Model file for the job. Use its own axes, mm. Coordinates: 2 decimals unless noted, no trailing zeros. Write each loop counter-clockwise with the first axis right and the second up, starting at its lowest first coordinate (ties: lowest second). Pieces come first, ordered by that corner, then holes. Notation, with made-up numbers: M -40,39 L 2,39 A31 cw 2,71 Z; hole C -31,-31 d1. An arc over 180 degrees is marked long. Answer in a Markdown table with one row per item. Add a question column.
```python
from build123d import *

# Parameters (mm, degrees)
SKETCH1_W               = 10
SKETCH1_H               = 10
PLATE_DEPTH             = 0.5
SKETCH2_R               = 0.2
ROD_DEPTH               = 0.25
LPATTERN1_COUNT         = 10
LPATTERN1_PITCH         = 1
LPATTERN1_COUNT_DIR2    = 10
LPATTERN1_PITCH_DIR2    = 1
BOSS_EXTRUDE3_DEPTH     = 0.5
SKETCH5_R               = 1.455938962
CUT_EXTRUDE1_DEPTH      = 0.5
CUT_EXTRUDE1_DEPTH_BACK = 1.5


with BuildPart() as part:
    # Sketch1 → Plate (new body)
    with BuildSketch(Plane(origin=(0, 0, 0), x_dir=(1, 0, 0), z_dir=(0, 1, 0))):
        Rectangle(SKETCH1_W, SKETCH1_H)
    extrude(amount=PLATE_DEPTH)

    # Sketch2 → Rod (add)
    with BuildSketch(Plane(origin=(0, 0.5, 0), x_dir=(1, 0, 0), z_dir=(0, 1, 0))):
        with Locations((-4.5, -4.5)):
            Circle(SKETCH2_R)
    rod = extrude(amount=ROD_DEPTH)

    # LPattern1: Rod 10 × 10
    with Locations(*[(i * LPATTERN1_PITCH, 0, -j * LPATTERN1_PITCH_DIR2) for i in range(LPATTERN1_COUNT) for j in range(LPATTERN1_COUNT_DIR2) if (i, j) != (0, 0)]):
        add(rod)

    # Sketch4 → Boss-Extrude3 (add)
    with BuildSketch(Plane(origin=(0, 0, 0), x_dir=(1, 0, 0), z_dir=(0, 1, 0))):
        with BuildLine():
            Line((-2, 7), (-2, 5))
            Line((-2, 5), (2, 5))
            Line((2, 5), (2, 7))
            ThreePointArc((2, 7), (0, 9), (-2, 7))
        make_face()
    extrude(amount=BOSS_EXTRUDE3_DEPTH)

    # Sketch5 → Cut-Extrude1 (cut, two sides)
    with BuildSketch(Plane(origin=(0, 0.5, 0), x_dir=(1, 0, 0), z_dir=(0, 1, 0))) as cut_extrude1_sk:
        with Locations((0, 7)):
            Circle(SKETCH5_R)
    extrude(amount=CUT_EXTRUDE1_DEPTH, mode=Mode.SUBTRACT)
    extrude(cut_extrude1_sk.sketch, amount=-CUT_EXTRUDE1_DEPTH_BACK, mode=Mode.SUBTRACT)


solid = part.part
```
1) Two-plate mould, pull along X, no slides. Class faces 1 (the face through (0.78, 0.25, -8.23)), 2 (the face through (0, 0.2, -9)), 3 (the face through (0, 0, -1)): released by +X, released by -X, zero draft, split by the parting line, or undercut.
2) Slice it at A-A (y = 0.25). Give the cut face in (x, z), then the cut area to 3 significant figures.
3) Flat gauge pin, fed straight in: pin 1 Ø1 at (x, z) = (-3, 2.5) entering from -Y. Where does the tip first touch, or does it go through?
4) Slice it at C-C (z = 0). Give the cut face in (x, y), then the cut area to 3 significant figures.
5) Drill centre lines: probe 1 along X at (y, z) = (0.15, -7); probe 2 along Z at (x, y) = (0, 0.2); probe 3 along Y at (x, z) = (-1.25, 3.5). Where is each one in solid material? Low to high.
6) Slice it at B-B (z = -8). Give the cut face in (x, y).
Ans:
| question | item | result |
|---|---|---|
| 1 | face 1 | undercut |
| 1 | face 2 | split by the parting line |
| 1 | face 3 | zero draft |
| 2 | outline | M -5,-5 L -2,-5 L -2,-7 A2 ccw 2,-7 L 2,-5 L 5,-5 L 5,5 L -5,5 Z; hole C 0,-7 d2.91 |
| 2 | area | 108 mm2 |
| 3 | pin 1 | stops at y = 0 |
| 4 | outline | M -5,0 L 5,0 L 5,0.5 L -5,0.5 Z |
| 4 | area | 5.00 mm2 |
| 5 | probe 1 | x = -2 to -1.46, 1.46 to 2 |
| 5 | probe 2 | z = -9 to -8.46, -5.54 to 5 |
| 5 | probe 3 | y = 0 to 0.5 |
| 6 | outline | M -1.73,0 L -1.06,0 L -1.06,0.5 L -1.73,0.5 Z; M 1.06,0 L 1.73,0 L 1.73,0.5 L 1.06,0.5 Z |
